Verification items for this drawing (mm, ordinates from the low corner). Give positions to 0.01 mm unless a question says otherwise; leave off trailing zeros. Loops run counter-clockwise (first coordinate to the right, second up) from the corner with the lowest first, then second, coordinate; pieces in that order, holes last. Notation, with made-up numbers: (-28.75, 0.25) - (-14.75, 0.25) arc R22 cw to (-14.75, 25.25) - close; hole circle Ø6 at (8.5, 61). An arc over 180 degrees is marked (long way). One line per question, with ' | ' between items. Start each with the question number.
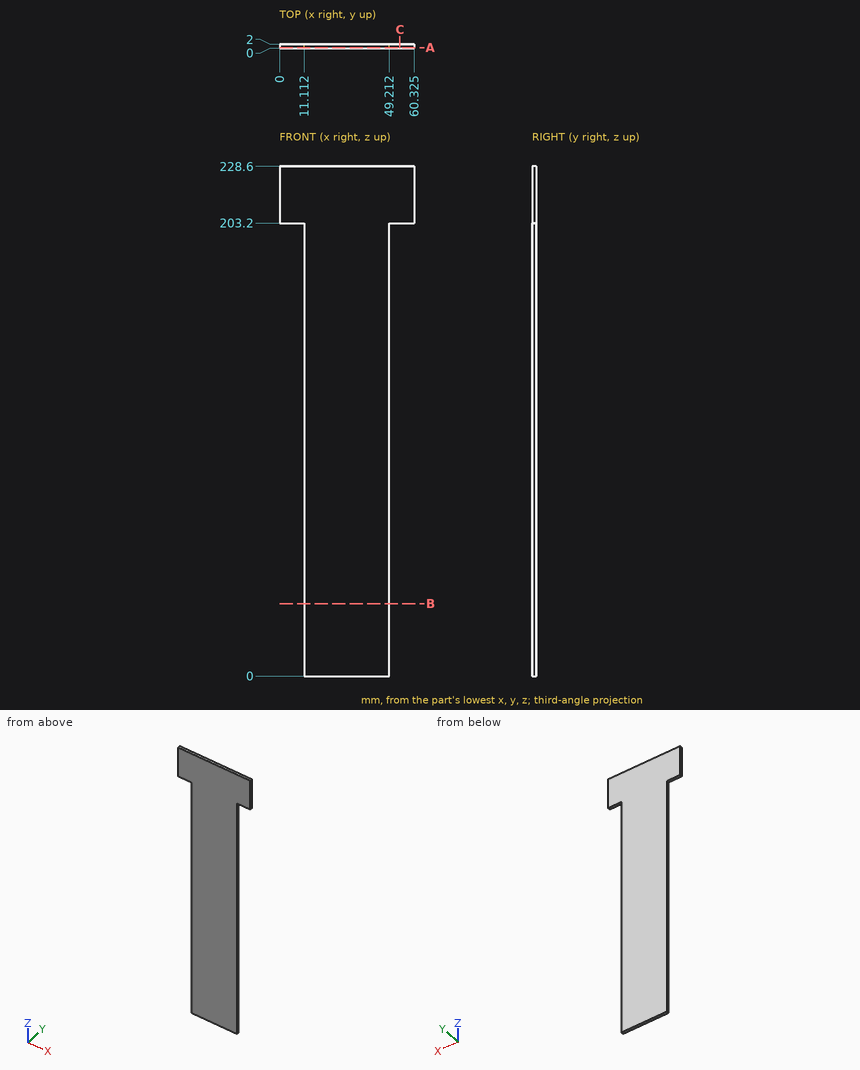
(1) Section check A-A, the plane y = 0.35. Record the boundary of the cut face in (x, z) (1 decimal).
(2) Section check C-C, the plane x = 54. Record the boundary of the cut face in (y, z).
(3) Material ranges on line 1 (Z direction, x = 54, y = 0.95); line 2 (X direction, y = 1.25, z = 42.5), recorded low to high.
(4) Depth check by flat-ended pin: pin 1 Ø0.6 at (x, y) = (6.5, 1) entering from -Z; pin 2 Ø0.6 at (y, z) = (1, 83.5) entering from -X. Enter the tip coordinate at first touch or a pass-through.
(5) Section check B-B, the plane z = 32.5. Record the boundary of the cut face in (x, y).
Numbers:
1) outline: (0, 203.2) - (11.1, 203.2) - (11.1, 0) - (49.2, 0) - (49.2, 203.2) - (60.3, 203.2) - (60.3, 228.6) - (0, 228.6) - close
2) outline: (0, 203.2) - (2, 203.2) - (2, 228.6) - (0, 228.6) - close
3) line 1: 203.2 to 228.6 | line 2: 11.11 to 49.21
4) pin 1: z = 203.2 | pin 2: x = 11.11
5) outline: (11.11, 0) - (49.21, 0) - (49.21, 2) - (11.11, 2) - close
